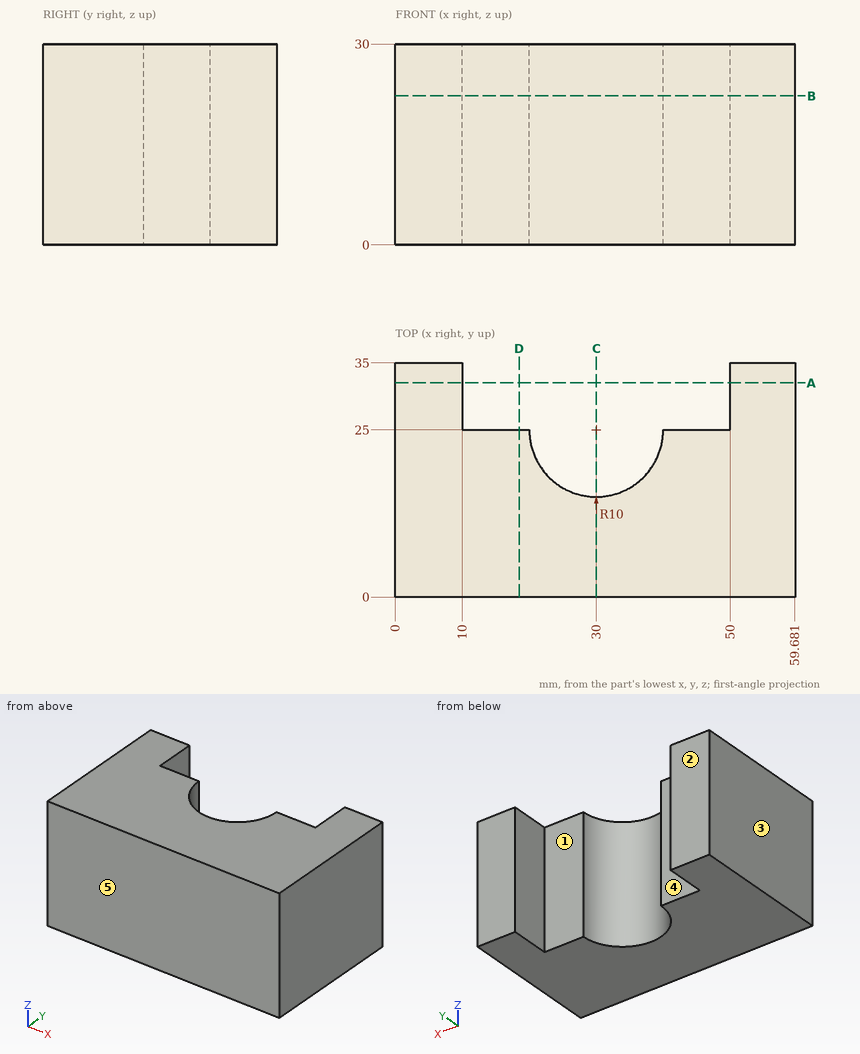
For this review, use the dimensioned drawing (mm, ordinates from the lowest corner) and the shaded views. A direction names the side the tool comes from. Round coordinates to 2 decimals unless told otherwise and drop trailing zeros. Write each loop counter-clockwise with the first axis right and the second up, starting at its lowest first coordinate (ties: lowest second). Pieces come first, ordered by that corner, then holes. Notation, with made-up numbers: (77, 69) - (121, 69) arc R19 ccw to (121, 95) - close; hole circle Ø11 at (12, 7). An arc over 180 degrees is marked (long way). Use a Markdown table: item, result.
Q1. The part is to be moulded in two halves that separate along X. For the marked faces 1, 2 and 3, say which applies: pulls with the +X half, pulls with the -X half, needs draft (parallel to the pull), parting line crosses it, or undercut.
Derived:
| item | result |
|---|---|
| face 1 | undercut |
| face 2 | needs draft |
| face 3 | pulls with the -X half |
Q2. We need section A-A (y = 32). Give the boundary of the cut face in (x, z).
Derived:
| item | result |
|---|---|
| outline | (0, 0) - (10, 0) - (10, 30) - (0, 30) - close; (50, 0) - (59.68, 0) - (59.68, 30) - (50, 30) - close |
Q3. Clearance check with a flat-ended pin moving along its axis: pin 1 (5 mm diameter, centred on x = 44, z = 7.5, fed in from +Y). State where the tip first meets the part, or that it passes through.
Derived:
| item | result |
|---|---|
| pin 1 | stops at y = 25 |
Q4. Machinability: for the marked faces 4 and 5, which of the approach directions +Z, -Z, +X, -X, +Y, -Y give a long, thin tool a straight path to every point of the face, cutting with its end or side? Answer none if there is none.
Derived:
| item | result |
|---|---|
| face 4 | +Z, -Z, +Y |
| face 5 | +Z, -Z, +X, -X, -Y |
Q5. We need section D-D (x = 18.5). Give the boundary of the cut face in (y, z).
Derived:
| item | result |
|---|---|
| outline | (0, 0) - (25, 0) - (25, 30) - (0, 30) - close |
Q6. We need section C-C (x = 30). Give the boundary of the cut face in (y, z).
Derived:
| item | result |
|---|---|
| outline | (0, 0) - (15, 0) - (15, 30) - (0, 30) - close |
Q7. We need section B-B (z = 22.25). Give the boundary of the cut face in (x, y).
Derived:
| item | result |
|---|---|
| outline | (0, 0) - (59.68, 0) - (59.68, 35) - (50, 35) - (50, 25) - (40, 25) arc R10 cw to (20, 25) - (10, 25) - (10, 35) - (0, 35) - close |
Q8. Wall thickness on line 1 along X through (y, z) = (27, 7.25); line 2 along X through (y, z) = (24.5, 22.75); line 3 along Y through (x, z) = (12.5, 25.25): over which ranges is each line inside the solid? List them lowest first.
Derived:
| item | result |
|---|---|
| line 1 | x = 0 to 10, 50 to 59.68 |
| line 2 | x = 0 to 20.01, 39.99 to 59.68 |
| line 3 | y = 0 to 25 |
